Check sheet for the modelled part. Datum: model origin and axes. Units: mm. A direction names the side the tool comes from. Round coordinates to 2 decimals unless told otherwise and drop trailing zeros. Order: outer loops, then holes, each group sorted by start corner. A loop starts at its lowest first (then second) coordinate and runs counter-clockwise, first axis right, second up. Notation, with made-up numbers: (28, 62) -> (42, 62) arc R21 ccw to (42, 72) -> close; hole circle Ø11 at (19, 50). An arc over 180 degrees is marked (long way). Answer in a Markdown table with one row per item.
from build123d import *

# Parameters (mm, degrees)
PAD_DEPTH       = 10
SKETCH001_W     = 10
SKETCH001_H     = 4
SKETCH001_W_2   = 15
SKETCH001_H_2   = 5.5
SKETCH001_W_3   = 9
SKETCH001_H_3   = 5
SKETCH001_W_4   = 14
SKETCH001_H_4   = 16.5
SKETCH001_W_5   = 16
SKETCH001_H_5   = 16
SKETCH001_W_6   = 17
POCKET_DEPTH    = 1
SKETCH002_R     = 12
POCKET001_DEPTH = 9
SKETCH003_W     = 41
SKETCH003_H     = 19
POCKET002_DEPTH = 9
SKETCH004_W     = 35
SKETCH004_H     = 12.5
POCKET003_DEPTH = 9
SKETCH005_W     = 41
SKETCH005_H     = 21
POCKET004_DEPTH = 9
SKETCH006_W     = 14
SKETCH006_H     = 12
POCKET005_DEPTH = 9
POCKET006_DEPTH = 9
SKETCH010_W     = 31.5
SKETCH010_H     = 26.5
POCKET007_DEPTH = 5
SKETCH011_W     = 27
SKETCH011_H     = 10
POCKET008_DEPTH = 9


with BuildPart() as part:
    # Sketch → Pad (new body)
    with BuildSketch(Plane.XY):
        Polygon((113.242246, 7.136342), (-0.047754, 7.136342), (-26.28226, -14.428265), (-26.28226, -35.968265), (-19.26312, -51.681819), (1.360962, -57.138638), (104.980466, -56.818034), (126.692617, -27.88965), (126.692617, -10.44965), align=None)
    extrude(amount=PAD_DEPTH)

    # Sketch001 (on Face11 of Pad) → Pocket (cut)
    with BuildSketch(Plane.XY.offset(10)):
        with Locations((4.5, -19)):
            Rectangle(SKETCH001_W, SKETCH001_H)
        with Locations((4.5, -34)):
            Rectangle(SKETCH001_W, SKETCH001_H)
        with Locations((67.5, -45.25)):
            Rectangle(SKETCH001_W_2, SKETCH001_H_2)
        with Locations((67.5, -7.5)):
            Rectangle(SKETCH001_W_3, SKETCH001_H_3)
        with Locations((102.5, -25)):
            Rectangle(SKETCH001_W_4, SKETCH001_H_4)
        with Locations((30.5, -13.25)):
            Rectangle(SKETCH001_W_5, SKETCH001_H_5)
        with Locations((30.5, -40.25)):
            Rectangle(SKETCH001_W_5, SKETCH001_H_5)
        with Locations((67.5, -26.5)):
            Rectangle(SKETCH001_W_6, SKETCH001_H_2)
    extrude(amount=-POCKET_DEPTH, mode=Mode.SUBTRACT)

    # Sketch002 (on Face4 of Pocket) → Pocket001 (cut)
    with BuildSketch(Plane(origin=(0, 0, 0), x_dir=(1, 0, 0), z_dir=(0, 0, -1))):
        with Locations((30.5, 40.25)):
            Circle(SKETCH002_R)
        with Locations((30.5, 13.25)):
            Circle(SKETCH002_R)
    extrude(amount=-POCKET001_DEPTH, mode=Mode.SUBTRACT)

    # Sketch003 (on Face4 of Pocket001) → Pocket002 (cut)
    with BuildSketch(Plane(origin=(0, 0, 0), x_dir=(1, 0, 0), z_dir=(0, 0, -1))):
        with Locations((67.481461, 7.5)):
            Rectangle(SKETCH003_W, SKETCH003_H)
    extrude(amount=-POCKET002_DEPTH, mode=Mode.SUBTRACT)

    # Sketch004 (on Face4 of Pocket002) → Pocket003 (cut)
    with BuildSketch(Plane(origin=(0, 0, 0), x_dir=(1, 0, 0), z_dir=(0, 0, -1))):
        with Locations((67.501572, 26.486867)):
            Rectangle(SKETCH004_W, SKETCH004_H)
    extrude(amount=-POCKET003_DEPTH, mode=Mode.SUBTRACT)

    # Sketch005 (on Face4 of Pocket003) → Pocket004 (cut)
    with BuildSketch(Plane(origin=(0, 0, 0), x_dir=(1, 0, 0), z_dir=(0, 0, -1))):
        with Locations((67.486454, 45.259564)):
            Rectangle(SKETCH005_W, SKETCH005_H)
    extrude(amount=-POCKET004_DEPTH, mode=Mode.SUBTRACT)

    # Sketch006 (on Face4 of Pocket004) → Pocket005 (cut)
    with BuildSketch(Plane(origin=(0, 0, 0), x_dir=(1, 0, 0), z_dir=(0, 0, -1))):
        with Locations((4.502728, 34.011238)):
            Rectangle(SKETCH006_W, SKETCH006_H)
    extrude(amount=-POCKET005_DEPTH, mode=Mode.SUBTRACT)

    # Sketch009 (on Face4 of Pocket005) → Pocket006 (cut)
    with BuildSketch(Plane(origin=(0, 0, 0), x_dir=(1, 0, 0), z_dir=(0, 0, -1))):
        Polygon((90, 36.5), (96, 36.5), (96, 45), (107, 45), (107, 36.5), (113, 36.5), (113, 13.5), (107, 13.5), (107, 5), (96, 5), (96, 13.5), (90, 13.5), align=None)
    extrude(amount=-POCKET006_DEPTH, mode=Mode.SUBTRACT)

    # Sketch010 (on Face4 of Pocket005) → Pocket007 (cut)
    with BuildSketch(Plane(origin=(0, 0, 0), x_dir=(1, 0, 0), z_dir=(0, 0, -1))):
        with Locations((30.25, 40.25)):
            Rectangle(SKETCH010_W, SKETCH010_H)
        with Locations((30.25, 13.25)):
            Rectangle(SKETCH010_W, SKETCH010_H)
    extrude(amount=-POCKET007_DEPTH, mode=Mode.SUBTRACT)

    # Sketch011 (on Face4 of Pocket007) → Pocket008 (cut)
    with BuildSketch(Plane(origin=(0, 0, 0), x_dir=(1, 0, 0), z_dir=(0, 0, -1))):
        with Locations((4.5, 19)):
            Rectangle(SKETCH011_W, SKETCH011_H)
    extrude(amount=-POCKET008_DEPTH, mode=Mode.SUBTRACT)


solid = part.part
Item 1: Cross-section at D-D (y = -7). Record the boundary of the cut face in (x, z), and give its area (3 significant figures).
Result sheet:
| item | result |
|---|---|
| outline | (-17.25, 0) -> (14.5, 0) -> (14.5, 5) -> (20.26, 5) -> (20.26, 9) -> (22.5, 9) -> (22.5, 10) -> (-17.25, 10) -> close; (38.5, 9) -> (40.74, 9) -> (40.74, 5) -> (46, 5) -> (46, 0) -> (46.98, 0) -> (46.98, 9) -> (63, 9) -> (63, 10) -> (38.5, 10) -> close; (72, 9) -> (87.98, 9) -> (87.98, 0) -> (96, 0) -> (96, 9) -> (107, 9) -> (107, 0) -> (124.05, 0) -> (124.05, 10) -> (72, 10) -> close |
| area | 681 mm^2 |
Item 2: Cross-section at B-B (y = -46.5). Record the boundary of the cut face in (x, z), and give its area (3 significant figures).
Result sheet:
| item | result |
|---|---|
| outline | (-21.58, 0) -> (14.5, 0) -> (14.5, 5) -> (20.26, 5) -> (20.26, 9) -> (22.5, 9) -> (22.5, 10) -> (-21.58, 10) -> close; (38.5, 9) -> (40.74, 9) -> (40.74, 5) -> (46, 5) -> (46, 0) -> (46.99, 0) -> (46.99, 9) -> (60, 9) -> (60, 10) -> (38.5, 10) -> close; (75, 9) -> (87.99, 9) -> (87.99, 0) -> (112.72, 0) -> (112.72, 10) -> (75, 10) -> close |
| area | 704 mm^2 |
Item 3: Set-up check for faces 1 (the flat face through (-26.282, -25, 5)), 2 (the flat face through (46.986, -45, 4)): record each of +Z, -Z, +X, -X, +Y, -Y from which the full face is reachable in a straight line by a thin tool's end or side.
Result sheet:
| item | result |
|---|---|
| face 1 | +Z, -Z, -X, +Y, -Y |
| face 2 | -Z |
Item 4: Cross-section at A-A (x = 30.5). Record the boundary of the cut face in (y, z).
Result sheet:
| item | result |
|---|---|
| outline | (-57.05, 0) -> (-53.5, 0) -> (-53.5, 5) -> (-52.25, 5) -> (-52.25, 9) -> (-48.25, 9) -> (-48.25, 10) -> (-57.05, 10) -> close; (-32.25, 9) -> (-28.25, 9) -> (-28.25, 5) -> (-27, 5) -> (-27, 0) -> (-26.5, 0) -> (-26.5, 5) -> (-25.25, 5) -> (-25.25, 9) -> (-21.25, 9) -> (-21.25, 10) -> (-32.25, 10) -> close; (-5.25, 9) -> (-1.25, 9) -> (-1.25, 5) -> (0, 5) -> (0, 0) -> (7.14, 0) -> (7.14, 10) -> (-5.25, 10) -> close |
Item 5: Mould release check, pull along X, two halves, no side actions. Record for faces 3 (the flat face through (67, -20.237, 4)), 4 (the flat face through (-12.981, -3.495, 4.93)), 5 (the flat face through (115.68, -42.56, 4.93)): pulls with the +X half, pulls with the -X half, needs draft (parallel to the pull), parting line crosses it, or undercut.
Result sheet:
| item | result |
|---|---|
| face 3 | undercut |
| face 4 | pulls with the -X half |
| face 5 | pulls with the +X half |
Item 6: Depth check by flat-ended pin: P1, Ø1.1, axis at y = -8, z = 9.5, coming from the -X side; P2, Ø0.5, axis at y = -11.5, z = 9.5, coming from the -X side; P3, Ø6, axis at x = 86.5, z = 5, coming from the -Y side; P4, Ø1, axis at x = 93, y = -42.5, coming from the -Z side. Enter the tip coordinate at first touch or a pass-through.
Result sheet:
| item | result |
|---|---|
| P1 | stops at x = -19.13 |
| P2 | stops at x = -23.02 |
| P3 | stops at y = -56.88 |
| P4 | stops at z = 0 |
Item 7: Cross-section at C-C (z = 2.75). State how many separate pieces and enclosed holes the cut face has, and give its area (3 significant figures).
Result sheet:
| item | result |
|---|---|
| separate pieces | 1 |
| enclosed holes | 7 |
| area | 4,080 mm^2 |
Item 8: Scan lines: line 1 (Y direction, x = 11, z = 8.5); line 2 (X direction, y = -22, z = 4.5); line 3 (X direction, y = -50.5, z = 3.5). Record each from-to range of solid material in increasing order. Write a range as [from, to].
Result sheet:
| item | result |
|---|---|
| line 1 | y = [-57.11, -40.01], [-28.01, -24], [-14, 7.14] |
| line 2 | x = [-26.28, -9], [46, 50], [85, 90], [113, 126.69] |
| line 3 | x = [-19.79, 14.5], [46, 46.99], [87.99, 109.72] |
